from build123d import *

# Parameters (mm, degrees)
F1_DEPTH = 11.8618
F2_W     = 97.282
F2_H     = 7.874
F3_DEPTH = 5.842
F4_W     = 2.286
F4_H     = 7.874
F5_DEPTH = 6.35


with BuildPart() as f1:
    # F0 (on Top) → F1 (new body)
    with BuildSketch(Plane.XY):
        Polygon((-120.65, 0), (0, 0), (0, 165.1), align=None)
    extrude(amount=F1_DEPTH)

    # F2 (on face) → F3 (join)
    with BuildSketch(Plane.XZ):
        with Locations((-54.229, 5.9309)):
            Rectangle(F2_W, F2_H)
    extrude(amount=F3_DEPTH)

    # F4 (on face) → F5 (join)
    with BuildSketch(Plane.XZ):
        with Locations((-3.41022, 5.9309)):
            Rectangle(F4_W, F4_H)
    extrude(amount=F5_DEPTH)


solid = f1.part
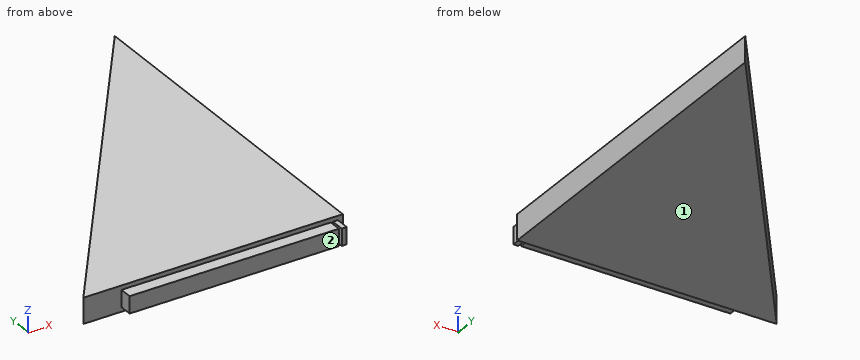
Design review of the part built by this model. Coordinates are the model's own, in mm. Face numbers are marked on the shaded views. A direction names the side the tool comes from. Give positions to 0.01 mm unless a question says otherwise; leave off trailing zeros. Loops run counter-clockwise (first coordinate to the right, second up) from the corner with the lowest first, then second, coordinate; pieces in that order, holes last. Notation, with made-up numbers: (51.25, -36) - (98.25, -36) arc R30 ccw to (98.25, -9) - close; hole circle Ø9 at (-22, -18.75). An arc over 180 degrees is marked (long way). Write item = value, one per line.
1) Clearance check with flat-ended pins moving along their axes: pin 1 Ø4.5 at (x, y) = (-66.5, -3) entering from +Z; pin 2 Ø3 at (y, z) = (-3.5, 5.5) entering from +X; pin 3 Ø1 at (x, z) = (-41.5, 5.5) entering from +Y. State where each tip first meets the part, or that it passes through.
Result sheet:
pin_1 = 9.87
pin_2 = -2.27
pin_3 = 108.99
2) Tool access review of the marked faces 1 and 2: name each direction out of +Z, -Z, +X, -X, +Y, -Y from which nothing blocks a thin tool from reaching the whole face with its end or side.
Result sheet:
face_1 = -Z, +X, -X, +Y, -Y
face_2 = +Z, -Z, -X, -Y
3) To check wall thickness, follow line 1 (X direction, y = 17, z = 2.5); line 2 (Y direction, x = -99, z = 9); line 3 (X direction, y = 128, z = 6.5). State the ranges of each line that lie inside material, in increasing order.
Result sheet:
line_1 = -108.23 to 0
line_2 = -5.84 to 29.63
line_3 = -27.11 to 0
4) Take a section at D-D on x = -62.5. State the section outline as (y, z) points, and give its area (3 significant figures).
Result sheet:
outline = (-5.84, 1.99) - (0, 1.99) - (0, 0) - (79.57, 0) - (79.57, 11.86) - (0, 11.86) - (0, 9.87) - (-5.84, 9.87) - close
area = 990 mm2
5) Take a section at B-B on x = -8. State the section outline as (y, z) points, and give its area (3 significant figures).
Result sheet:
outline = (-5.84, 1.99) - (0, 1.99) - (0, 0) - (154.15, 0) - (154.15, 11.86) - (0, 11.86) - (0, 9.87) - (-5.84, 9.87) - close
area = 1,870 mm2
6) Take a section at C-C on y = 21. State the section outline as (x, z) points.
Result sheet:
outline = (-105.3, 0) - (0, 0) - (0, 11.86) - (-105.3, 11.86) - close
7) Take a section at A-A on z = 6.25. State the section outline as (x, y) points.
Result sheet:
outline = (-120.65, 0) - (-102.87, 0) - (-102.87, -5.84) - (-5.59, -5.84) - (-5.59, 0) - (-4.55, 0) - (-4.55, -6.35) - (-2.27, -6.35) - (-2.27, 0) - (0, 0) - (0, 165.1) - close
